Design review of the part built by this model. Coordinates are the model's own, in mm. Give positions to 0.01 mm unless a question says otherwise; leave off trailing zeros. Order: outer loops, then holes, each group sorted by start corner. A loop starts at its lowest first (then second) coordinate and runs counter-clockwise, first axis right, second up.
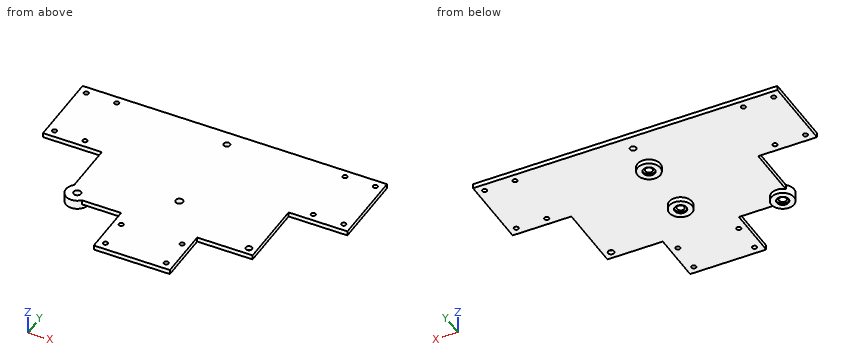
```python
from build123d import *

# Parameters (mm, degrees)
ESQUISSE1_R             = 2
ESQUISSE1_R_2           = 1.5
BOSS_EXTRU_1_DEPTH      = 3
BOSS_EXTRU_2_START      = -3
ESQUISSE3_R             = 7.5
BOSS_EXTRU_2_DEPTH      = 6
ESQUISSE4_R             = 3.875
ENL_V_MAT_EXTRU_1_DEPTH = 1
ESQUISSE5_R             = 2.375
ENL_V_MAT_EXTRU_2_DEPTH = 4
ENL_V_MAT_EXTRU_3_REACH = 3
ESQUISSE6_R             = 2.375


with BuildPart() as part:
    # Esquisse1 → Boss.-Extru.1 (new body)
    with BuildSketch(Plane.XY):
        Polygon((0, 50), (-100, 50), (-100, 0), (-61.381557247, 0), (-61.381557247, -45.5212086), (-25, -45.5212086), (-25, -80), (25, -80), (25, -45.5212086), (61.381557247, -45.5212086), (61.381557247, 0), (100, 0), (100, 50), align=None)
        with Locations((0, 20)):
            Circle(ESQUISSE1_R, mode=Mode.SUBTRACT)
        with Locations((0, -20)):
            Circle(ESQUISSE1_R, mode=Mode.SUBTRACT)
        with Locations((0, 40)):
            Circle(ESQUISSE1_R, mode=Mode.SUBTRACT)
        with Locations((-20, -55)):
            Circle(ESQUISSE1_R_2, mode=Mode.SUBTRACT)
        with Locations((20, -55)):
            Circle(ESQUISSE1_R_2, mode=Mode.SUBTRACT)
        with Locations((20, -75)):
            Circle(ESQUISSE1_R_2, mode=Mode.SUBTRACT)
        with Locations((-20, -75)):
            Circle(ESQUISSE1_R_2, mode=Mode.SUBTRACT)
        with Locations((-95, 45)):
            Circle(ESQUISSE1_R_2, mode=Mode.SUBTRACT)
        with Locations((-75, 45)):
            Circle(ESQUISSE1_R_2, mode=Mode.SUBTRACT)
        with Locations((-75, 5)):
            Circle(ESQUISSE1_R_2, mode=Mode.SUBTRACT)
        with Locations((-95, 5)):
            Circle(ESQUISSE1_R_2, mode=Mode.SUBTRACT)
        with Locations((75, 5)):
            Circle(ESQUISSE1_R_2, mode=Mode.SUBTRACT)
        with Locations((95, 5)):
            Circle(ESQUISSE1_R_2, mode=Mode.SUBTRACT)
        with Locations((75, 45)):
            Circle(ESQUISSE1_R_2, mode=Mode.SUBTRACT)
        with Locations((95, 45)):
            Circle(ESQUISSE1_R_2, mode=Mode.SUBTRACT)
        with Locations((56.381557247, -40.5212086)):
            Circle(ESQUISSE1_R, mode=Mode.SUBTRACT)
        with Locations((-56.381557247, -40.5212086)):
            Circle(ESQUISSE1_R, mode=Mode.SUBTRACT)
    extrude(amount=BOSS_EXTRU_1_DEPTH)

    # Esquisse3 → Boss.-Extru.2 (add)
    with BuildSketch(Plane(origin=(0, 0, 0), x_dir=(-1, 0, 0), z_dir=(0, 0, -1)).offset(BOSS_EXTRU_2_START)):
        with Locations((0, 20)):
            Circle(ESQUISSE3_R)
        with Locations((56.381557247, -40.5212086)):
            Circle(ESQUISSE3_R)
        with Locations((0, -20)):
            Circle(ESQUISSE3_R)
    extrude(amount=BOSS_EXTRU_2_DEPTH)

    # Esquisse4 → Enlèv. mat.-Extru.1 (cut)
    with BuildSketch(Plane(origin=(0, 0, -3), x_dir=(-1, 0, 0), z_dir=(0, 0, -1))):
        with Locations((56.381557247, -40.5212086)):
            Circle(ESQUISSE4_R)
        with Locations((0, 20)):
            Circle(ESQUISSE4_R)
        with Locations((0, -20)):
            Circle(ESQUISSE4_R)
    extrude(amount=-ENL_V_MAT_EXTRU_1_DEPTH, mode=Mode.SUBTRACT)

    # Esquisse5 → Enlèv. mat.-Extru.2 (cut)
    with BuildSketch(Plane(origin=(0, 0, -2), x_dir=(-1, 0, 0), z_dir=(0, 0, -1))):
        with Locations((56.381557247, -40.5212086)):
            Circle(ESQUISSE5_R)
        with Locations((0, 20)):
            Circle(ESQUISSE5_R)
        with Locations((0, -20)):
            Circle(ESQUISSE5_R)
    extrude(amount=-ENL_V_MAT_EXTRU_2_DEPTH, mode=Mode.SUBTRACT)

    # Esquisse6 → Enlèv. mat.-Extru.3 (cut, up to next)
    with BuildSketch(Plane(origin=(0, 0, 2), x_dir=(-1, 0, 0), z_dir=(0, 0, -1)), mode=Mode.PRIVATE) as enl_v_mat_extru_3_sk1:
        with Locations((56.381557247, -40.5212086)):
            Circle(ESQUISSE6_R)
    enl_v_mat_extru_3_tool1 = extrude(enl_v_mat_extru_3_sk1.sketch, amount=-ENL_V_MAT_EXTRU_3_REACH, mode=Mode.PRIVATE) & part.part
    add(enl_v_mat_extru_3_tool1.solids().sort_by_distance((-56.381557, -40.521209, 2))[0], mode=Mode.SUBTRACT)
    # Esquisse6 → Enlèv. mat.-Extru.3 (cut, up to next)
    with BuildSketch(Plane(origin=(0, 0, 2), x_dir=(-1, 0, 0), z_dir=(0, 0, -1)), mode=Mode.PRIVATE) as enl_v_mat_extru_3_sk2:
        with Locations((0, -20)):
            Circle(ESQUISSE6_R)
    enl_v_mat_extru_3_tool2 = extrude(enl_v_mat_extru_3_sk2.sketch, amount=-ENL_V_MAT_EXTRU_3_REACH, mode=Mode.PRIVATE) & part.part
    add(enl_v_mat_extru_3_tool2.solids().sort_by_distance((0, -20, 2))[0], mode=Mode.SUBTRACT)


solid = part.part
```
1. Take a section at B-B (x = 0). State how many separate pieces and enclosed holes the cut face has, then the cut area to 3 significant figures.
Recorded:
separate pieces: 3
enclosed holes: 0
area: 410 mm2
2. For pin 1 (4.5 mm diameter, centred on x = 0, y = 40, fed in from -Z); pin 2 (1.4 mm diameter, centred on x = -0.5, y = 20.5, fed in from -Z); pin 3 (1.8 mm diameter, centred on x = 95, y = 45, fed in from +Z); pin 4 (0.9 mm diameter, centred on y = -63, z = 1.5, fed in from +X), all flat-tipped, find the tip position at first contact; note any pin that passes through.
Recorded:
pin 1: stops at z = 0
pin 2: stops at z = 2
pin 3: passes through
pin 4: stops at x = 25
3. For line 1 along Y through (x, z) = (-20, 0.85); line 2 along Y through (x, z) = (95, 1.05); line 3 along X through (y, z) = (-75, 1), list the stretches that pass through material, from the lowest coordinate up.
Recorded:
line 1: y = -80 to -76.5, -73.5 to -56.5, -53.5 to 50
line 2: y = 0 to 3.5, 6.5 to 43.5, 46.5 to 50
line 3: x = -25 to -21.5, -18.5 to 18.5, 21.5 to 25
4. Take a section at D-D (x = -28.5). State the section outline as (y, z) points.
Recorded:
outline: (-45.52, 0) - (50, 0) - (50, 3) - (-45.52, 3) - close
5. Take a section at C-C (y = 20). State the section outline as (x, z) points (3 decimals), then the cut area to 3 significant figures.
Recorded:
outline: (-100, 0) - (-7.5, 0) - (-7.5, -3) - (-3.875, -3) - (-3.875, -2) - (-2.375, -2) - (-2.375, 2) - (2.375, 2) - (2.375, -2) - (3.875, -2) - (3.875, -3) - (7.5, -3) - (7.5, 0) - (100, 0) - (100, 3) - (-100, 3) - close
area: 618 mm2
6. Take a section at A-A (y = 40). State the section outline as (x, z) points, then the cut area to 3 significant figures.
Recorded:
outline: (-100, 0) - (-2, 0) - (-2, 3) - (-100, 3) - close; (2, 0) - (100, 0) - (100, 3) - (2, 3) - close
area: 588 mm2
